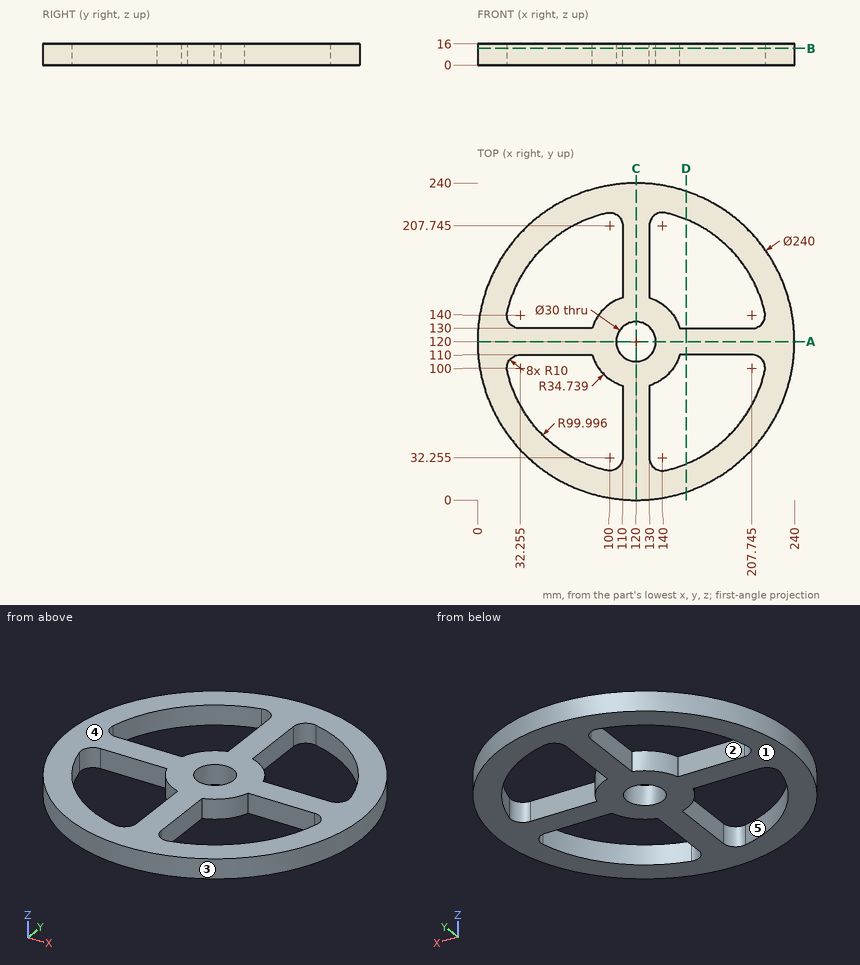
Check sheet for the drawn part. Datum: minimum x, y, z corner. Units: mm. A direction names the side the tool comes from. Round coordinates to 2 decimals unless told otherwise and drop trailing zeros. Loops run counter-clockwise (first coordinate to the right, second up) from the corner with the lowest first, then second, coordinate; pieces in that order, holes last.
Item 1: Thickness scan on line 1 (Y direction, x = 155.5, z = 5.75); line 2 (Y direction, x = 120, z = 10); line 3 (X direction, y = 189.5, z = 14.5) (1 decimal). Record the ranges inside material, lowest first.
Item 2: Access from +Z, -Z, +X, -X, +Y, -Y to the whole of each face (thin tool, end or side, straight path). Record for the marked faces 4 and 5.
Item 3: Gauge pin test, flat ends, axial feed: pin 1 (5 mm diameter, centred on y = 178, z = 6, fed in from +X) (1 decimal); pin 2 (5 mm diameter, centred on x = 48, z = 7.5, fed in from -Y) (1 decimal); pin 3 (8 mm diameter, centred on x = 83, z = 7.5, fed in from -Y). Record the tip position at first contact, or that the pin passes through.
Item 4: Cross-section at D-D on x = 158. Record the boundary of the cut face in (y, z) (1 decimal).
Item 5: Cross-section at A-A on y = 120. Record the boundary of the cut face in (x, z), then the cut area to 3 significant figures.
Item 6: Mould release check, pull along Y, two halves, no side actions. Record for the marked faces 1, 2 and 3: pulls with the +Y half, pulls with the -Y half, needs draft (parallel to the pull), parting line crosses it, or undercut.
Item 7: Cross-section at B-B on z = 12.75. Record the boundary of the cut face in (x, y) (1 decimal), then the cut area to 3 significant figures.
Answer sheet:
1. line 1: y = 5.37 to 26.52, 110 to 130, 213.48 to 234.63
1. line 2: y = 0 to 105, 135 to 240
1. line 3: x = 22.2 to 48.1, 110 to 130, 191.9 to 217.8
2. face 4: +Z, +X, -X, +Y, -Y
2. face 5: +Z, -Z
3. pin 1: stops at x = 226.4
3. pin 2: stops at y = 22.2
3. pin 3: stops at y = 4.63
4. outline: (6.2, 0) - (27.5, 0) - (27.5, 16) - (6.2, 16) - close; (110, 0) - (130, 0) - (130, 16) - (110, 16) - close; (212.5, 0) - (233.8, 0) - (233.8, 16) - (212.5, 16) - close
5. outline: (0, 0) - (105, 0) - (105, 16) - (0, 16) - close; (135, 0) - (240, 0) - (240, 16) - (135, 16) - close
5. area: 3,360 mm2
6. face 1: needs draft
6. face 2: undercut
6. face 3: parting line crosses it
7. outline: circle Ø240 at (120, 120); hole (22.5, 97.8) arc R100 ccw to (97.8, 22.5) arc R10 ccw to (110, 32.3) - (110, 86.7) arc R34.7 cw to (86.7, 110) - (32.3, 110) arc R10 ccw to start; hole (22.5, 142.2) arc R10 ccw to (32.3, 130) - (86.7, 130) arc R34.7 cw to (110, 153.3) - (110, 207.7) arc R10 ccw to (97.8, 217.5) arc R100 ccw to start; hole circle Ø30 at (120, 120); hole (130, 32.3) arc R10 ccw to (142.2, 22.5) arc R100 ccw to (217.5, 97.8) arc R10 ccw to (207.7, 110) - (153.3, 110) arc R34.7 cw to (130, 86.7) - close; hole (130, 153.3) arc R34.7 cw to (153.3, 130) - (207.7, 130) arc R10 ccw to (217.5, 142.2) arc R100 ccw to (142.2, 217.5) arc R10 ccw to (130, 207.7) - close
7. area: 22,400 mm2
